Input: part model. Units: mm. Frame: model coordinates. Face numbers are marked on the shaded views. A direction names the side the tool comes from. Round coordinates to 2 decimals unless told otherwise and drop trailing zeros. Order: outer loops, then holes, each group sorted by start corner. A loop starts at its lowest first (then second) coordinate and runs counter-clockwise, first axis right, second up.
Item 1: First-contact query: pin 1 (3 mm diameter, centred on y = 4.5, z = -18.5, fed in from -X); pin 2 (15 mm diameter, centred on x = 7, z = -6, fed in from +Y); pin 3 (3 mm diameter, centred on x = -18.5, y = 3, fed in from -Z). Flat tips, straight axial feed; report the tip coordinate or a pass-through.
Item 2: Cut plane D-D on y = 2.5. Output: boundary loops of the cut face in (x, z).
Item 3: Cut plane A-A on y = 7.25. Output: boundary loops of the cut face in (x, z), then the cut area to 3 significant figures.
Item 4: Cut plane B-B on x = -0.5. Output: boundary loops of the cut face in (y, z), then the cut area to 3 significant figures.
Item 5: Reachability of the marked faces 1, 2 and 3 from +Z, -Z, +X, -X, +Y, -Y: full face, straight path, thin tool, end or side. Return the list, or none.
Item 6: Line query: L1, parallel to Y at x = 10, z = -2; L2, parallel to Z at x = -21.5, y = 6; L3, parallel to Z at x = -3.5, y = 2.5. Output: solid intervals per line, ascending.
Item 7: Cut plane C-C on x = 9. Output: boundary loops of the cut face in (y, z).
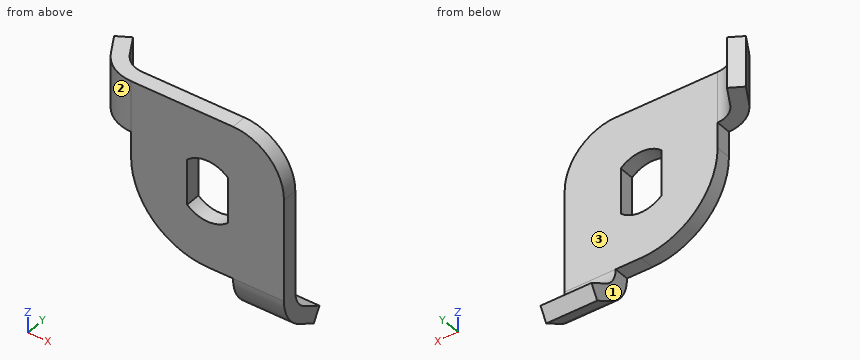
```python
from build123d import *

# Parameters (mm, degrees)
SKETCH1_W           = 30
SKETCH1_H           = 30
BOSS_EXTRUDE1_DEPTH = 3
BOSS_EXTRUDE2_DEPTH = 10
FILLET1_R           = 15
FILLET2_R           = 10
BOSS_EXTRUDE3_DEPTH = 10
CUT_EXTRUDE1_DEPTH  = 3


with BuildPart() as part:
    # Sketch1 → Boss-Extrude1 (new body)
    with BuildSketch(Plane(origin=(0, 0, 0), x_dir=(1, 0, 0), z_dir=(0, 1, 0))):
        Rectangle(SKETCH1_W, SKETCH1_H)
    extrude(amount=BOSS_EXTRUDE1_DEPTH)

    # Sketch2 → Boss-Extrude2 (add)
    with BuildSketch(Plane.XY.offset(15)):
        with BuildLine():
            Line((-21.580127019, 9.397114317), (-24.17820323, 7.897114317))
            Line((-24.17820323, 7.897114317), (-21.92820323, 4))
            ThreePointArc((-21.92820323, 4), (-19, 1.07179677), (-15, 0))
            Line((-15, 0), (-15, 3))
            ThreePointArc((-15, 3), (-17.5, 3.669872981), (-19.330127019, 5.5))
            Line((-19.330127019, 5.5), (-21.580127019, 9.397114317))
        make_face()
    extrude(amount=-BOSS_EXTRUDE2_DEPTH)

    # Fillet1
    fillet1_edges = [part.edges().sort_by_distance(p)[0] for p in [
        (-15, 1.5, -15),
    ]]
    fillet(fillet1_edges, radius=FILLET1_R)

    # Fillet2
    fillet2_edges = [part.edges().sort_by_distance(p)[0] for p in [
        (15, 1.5, 15),
    ]]
    fillet(fillet2_edges, radius=FILLET2_R)

    # Sketch3 → Boss-Extrude3 (add)
    with BuildSketch(Plane(origin=(15, 0, 0), x_dir=(0, 0, -1), z_dir=(1, 0, 0))):
        with BuildLine():
            Line((15, 3), (15, 0))
            ThreePointArc((15, 0), (19, 1.07179677), (21.92820323, 4))
            Line((21.92820323, 4), (24.17820323, 7.897114317))
            Line((24.17820323, 7.897114317), (21.580127019, 9.397114317))
            Line((21.580127019, 9.397114317), (19.330127019, 5.5))
            ThreePointArc((19.330127019, 5.5), (17.5, 3.669872981), (15, 3))
        make_face()
    extrude(amount=-BOSS_EXTRUDE3_DEPTH)

    # Sketch4 → Cut-Extrude1 (cut)
    with BuildSketch(Plane.XZ):
        with BuildLine():
            Line((-4, -4.472135955), (-4, 4.472135955))
            ThreePointArc((-4, 4.472135955), (0, 6), (4, 4.472135955))
            Line((4, 4.472135955), (4, -4.472135955))
            ThreePointArc((4, -4.472135955), (0, -6), (-4, -4.472135955))
        make_face()
    extrude(amount=-CUT_EXTRUDE1_DEPTH, mode=Mode.SUBTRACT)


solid = part.part
```
From the geometry:
1. pin 1: stops at x = 5
1. pin 2: stops at y = 3
1. pin 3: stops at z = 5
2. outline: (-20.81, 5) - (-15, 5) - (-15, 0) arc R15 ccw to (0, -15) - (5, -15) - (5, -20.81) - (15, -20.81) - (15, 5) arc R10 ccw to (5, 15) - (-20.81, 15) - close; hole (-4, -4.47) arc R6 ccw to (4, -4.47) - (4, 4.47) arc R6 ccw to (-4, 4.47) - close
3. outline: (-23.8, 5) - (-20.34, 5) - (-20.34, 15) - (-23.8, 15) - close; (5, -23.8) - (15, -23.8) - (15, -20.34) - (5, -20.34) - close
3. area: 69.3 mm2
4. outline: (0, -14.99) - (3, -14.99) - (3, -5.98) - (0, -5.98) - close; (0, 5.98) - (3, 5.98) - (3, 15) - (0, 15) - close
4. area: 54.1 mm2
5. face 1: -Z, -X, +Y, -Y
5. face 2: +Z, -Z, -X, -Y
5. face 3: +Z, +X, +Y
6. L1: y = 0 to 3
6. L2: z = 5 to 15
6. L3: z = -14.59 to -4.87, 4.87 to 15
7. outline: (0, -15) arc R8 ccw to (4, -21.93) - (7.9, -24.18) - (9.4, -21.58) - (5.5, -19.33) arc R5 cw to (3, -15) - (3, 14.17) - (0, 14.17) - close
